```python
from build123d import *

# Parameters (mm, degrees)
SKETCH1_R           = 4
SKETCH1_R_2         = 2
BOSS_EXTRUDE1_DEPTH = 2
CUT_EXTRUDE1_DEPTH  = 173.793238563


with BuildPart() as part:
    # Sketch1 → Boss-Extrude1 (new body)
    with BuildSketch(Plane.XY):
        Polygon((-12.69170221, 68.058974673), (-21.206087924, 61.497173254), (-26.925864701, 61.497173254), (-78.416756166, 95.875975746), (-89.405776689, 94.940877802), (-109.330638194, 108.244063256), (-110.106321881, 117.359690148), (-107.452090358, 123.920131464), (-102.997288795, 129.41913849), (-94.646003522, 133.154426043), (-73.358414132, 122.162911716), (-68.855470773, 112.095316109), (-13.842945112, 83.690457631), (-11.073314648, 78.685960307), align=None)
        with Locations((-90.332829692, 113.828343926)):
            Circle(SKETCH1_R, mode=Mode.SUBTRACT)
        with Locations((-18.448275862, 69.087716549)):
            Circle(SKETCH1_R_2, mode=Mode.SUBTRACT)
        with Locations((-32.842285033, 70.837716549)):
            Circle(SKETCH1_R_2, mode=Mode.SUBTRACT)
        with Locations((-31.39400917, 82.75)):
            Circle(SKETCH1_R_2, mode=Mode.SUBTRACT)
        with Locations((-17, 81)):
            Circle(SKETCH1_R_2, mode=Mode.SUBTRACT)
        Polygon((-102.715959344, 111.122206654), (-96.771854102, 112.676201947), (-96.173964404, 110.389245671), (-102.118069647, 108.835250378), align=None, mode=Mode.SUBTRACT)
        Polygon((-91.670790351, 126.557551491), (-90.152197928, 120.604303172), (-92.442671943, 120.0200345), (-93.961264367, 125.97328282), align=None, mode=Mode.SUBTRACT)
        Polygon((-77.94970004, 116.534481198), (-83.893805282, 114.980485905), (-84.49169498, 117.267442181), (-78.547589737, 118.821437474), align=None, mode=Mode.SUBTRACT)
        Polygon((-88.222987441, 107.636653352), (-90.513461456, 107.052384681), (-88.994869033, 101.099136361), (-86.704395017, 101.683405032), align=None, mode=Mode.SUBTRACT)
    extrude(amount=BOSS_EXTRUDE1_DEPTH)

    # Sketch5 → Cut-Extrude1 (cut, through all)
    with BuildSketch(Plane(origin=(0, 0, 0), x_dir=(-1, 0, 0), z_dir=(0, 0, -1))):
        Polygon((40.900602426, 76.238480364), (36.043275579, 90.088799545), (49.371469789, 96.970604475), align=None)
        Polygon((49.606538592, 82.051152303), (57.395163154, 101.113513236), (62.081526665, 90.380298271), align=None)
        Polygon((62.153457083, 103.570383994), (66.596381061, 93.394720495), (79.071369134, 101.723866464), align=None)
    extrude(amount=-CUT_EXTRUDE1_DEPTH, mode=Mode.SUBTRACT)


solid = part.part
```
Could you check a few things on this model? Use its own coordinates, in mm. A direction names the side the tool comes from. Round coordinates to 2 decimals unless told otherwise and drop trailing zeros. Write each loop counter-clockwise with the first axis right and the second up, starting at its lowest first coordinate (ties: lowest second). Pieces come first, ordered by that corner, then holes.
(1) If I drill on probe 1 along X at (y, z) = (93, 0.4); probe 2 along X at (y, z) = (111, 1.05); probe 3 along Y at (x, z) = (-34.5, 0.2), over which ranges is the centre line in solid material (lowest first)?
Findings below:
probe 1: x = -74.11 to -60.94, -54.08 to -47.75, -41.68 to -31.87
probe 2: x = -109.57 to -102.68, -96.33 to -93.16, -87.5 to -66.73
probe 3: y = 66.55 to 69.72, 71.96 to 94.36
(2) Suppose I cut it at D-D on y = 74.5. Write out the boundary of the cut face in (x, z), and give its area (3 significant figures).
Findings below:
outline: (-46.4, 0) - (-11.71, 0) - (-11.71, 2) - (-46.4, 2) - close
area: 69.4 mm2
(3) Suppose I cut it at A-A on y = 99. Write out the boundary of the cut face in (x, z), and give its area (3 significant figures).
Findings below:
outline: (-95.49, 0) - (-74.99, 0) - (-74.99, 2) - (-95.49, 2) - close; (-64.15, 0) - (-58.32, 0) - (-58.32, 2) - (-64.15, 2) - close; (-56.53, 0) - (-43.49, 0) - (-43.49, 2) - (-56.53, 2) - close
area: 78.7 mm2
(4) Suppose I cut it at B-B on x = -72. Write out the boundary of the cut face in (y, z), and give its area (3 significant figures).
Findings below:
outline: (91.59, 0) - (97, 0) - (97, 2) - (91.59, 2) - close; (102.5, 0) - (119.13, 0) - (119.13, 2) - (102.5, 2) - close
area: 44.1 mm2
(5) Suppose I cut it at C-C on z = 1.5. State how many separate pieces and enclosed holes the cut face has, and give its area (3 significant figures).
Findings below:
separate pieces: 1
enclosed holes: 12
area: 2,170 mm2
(6) Thinking about a two-plate mould opening in X: for faces 4 (the face through (-24, 61.497, 1)), 5 (the face through (-41.73, 98.09, 0.99)), 6 (the face through (-72.747, 97.501, 0.986)), which applies, +X half, -X half, draft (parallel to the pull), parting line (faces both ways), or undercut?
Findings below:
face 4: draft
face 5: +X half
face 6: undercut
(7) Which directions (+Z, -Z, +X, -X, +Y, -Y) give clear straight access to the entire face, cutting with the end or side of a thin tool? Please do faces 1 (the face through (-83.834, 95.415, 0.986)), 2 (the face through (-89.35, 107.35, 0.99)), 3 (the face through (-60, 100, 2)).
Findings below:
face 1: +Z, -Z, -Y
face 2: +Z, -Z
face 3: +Z, +X, -X, +Y, -Y
